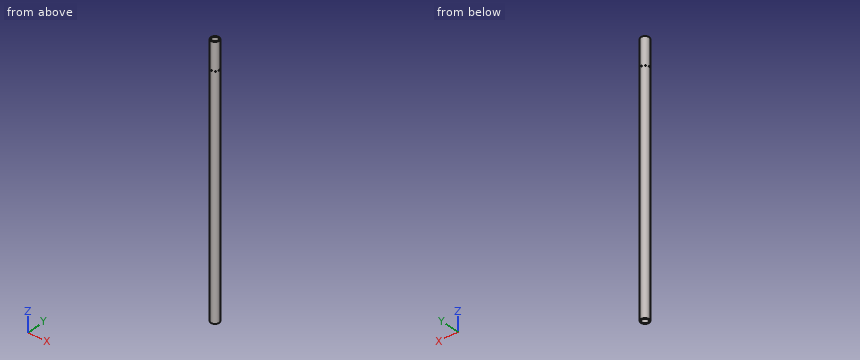
```python
from build123d import *

# Parameters (mm, degrees)
SKETCH_R           = 4
SKETCH_R_2         = 3
PAD_DEPTH          = 250
SKETCH001_W        = 5
SKETCH001_H        = 5
PAD001_DEPTH       = 10
SKETCH002_R        = 0.5
POCKET_DEPTH       = 3
POLARPATTERN_COUNT = 8
SKETCH003_W        = 8.429369
SKETCH003_H        = 7.155477
POCKET001_DEPTH    = 10


with BuildPart() as part:
    # Sketch → Pad (new body)
    with BuildSketch(Plane.XY.offset(44)):
        Circle(SKETCH_R)
        Circle(SKETCH_R_2, mode=Mode.SUBTRACT)
    extrude(amount=PAD_DEPTH)

    # Sketch001 → Pad001 (new body)
    with BuildSketch(Plane.XY.offset(294)):
        with Locations((2.5, -2.5)):
            Rectangle(SKETCH001_W, SKETCH001_H)
    extrude(amount=PAD001_DEPTH)

    # Sketch002 → Pocket (cut)
    with BuildSketch(Plane(origin=(0, -5, 44), x_dir=(1, 0, 0), z_dir=(0, -1, 0))):
        with Locations((0, 224)):
            Circle(SKETCH002_R)
    pocket = extrude(amount=-POCKET_DEPTH, mode=Mode.SUBTRACT)

    # PolarPattern: Pocket ×8 about axis
    polarpattern_axis = Axis((0, 0, 299), (0, 0, 1))
    for i in range(1, POLARPATTERN_COUNT):
        add(pocket.rotate(polarpattern_axis, i * 360 / POLARPATTERN_COUNT), mode=Mode.SUBTRACT)

    # Sketch003 → Pocket001 (cut)
    with BuildSketch(Plane.XY.offset(304)):
        with Locations((3.121665, -2.696092)):
            Rectangle(SKETCH003_W, SKETCH003_H)
    extrude(amount=-POCKET001_DEPTH, mode=Mode.SUBTRACT)


solid = part.part
```
The model under review builds one solid part; all positions refer to its coordinate system, in mm. Coordinates: 2 decimals unless noted, no trailing zeros. Write each loop counter-clockwise with the first axis right and the second up, starting at its lowest first coordinate (ties: lowest second). Pieces come first, ordered by that corner, then holes.
1) Clearance check with flat-ended pins moving along their axes: pin 1 Ø1.5 at (x, z) = (0.5, 257) entering from -Y; pin 2 Ø4 at (x, z) = (3, 255.5) entering from -Y; pin 3 Ø3 at (y, z) = (2.5, 166) entering from +X; pin 4 Ø3 at (x, y) = (-1, 1) entering from -Z. State where each tip first meets the part, or that it passes through.
2) We need section A-A on z = 251. State the section outline as (x, y) points, then the cut area to 3 significant figures.
3) To check wall thickness, follow probe 1 along Z at (x, y) = (0, -3.45); probe 2 along Y at (x, z) = (0, 104.5). State the ranges of each line that lie inside material, in increasing order.
Answer list:
1. pin 1: stops at y = -4
1. pin 2: stops at y = -3.87
1. pin 3: stops at x = 3.87
1. pin 4: passes through
2. outline: circle Ø8 at (0, 0); hole circle Ø6 at (0, 0)
2. area: 22.0 mm2
3. probe 1: z = 44 to 267.5, 268.5 to 294
3. probe 2: y = -4 to -3, 3 to 4
